Work out the finished part from the listing and answer in its coordinate system (mm). A direction names the side the tool comes from. Coordinates: 2 decimals unless noted, no trailing zeros. Loops run counter-clockwise (first coordinate to the right, second up) from the corner with the lowest first, then second, coordinate; pieces in that order, holes last. Notation, with made-up numbers: (70, -22.75) -> (84, -22.75) arc R24 ccw to (84, 7.25) -> close; hole circle Ø11 at (73.25, 47). An arc over 180 degrees is marked (long way). Answer as CSV lines item,"result".
```python
from build123d import *

# Parameters (mm, degrees)
DODANIE_WYCI_GNI_CIE1_DEPTH = 10
WYTNIJ_WYCI_GNI_CIE1_REACH  = 105.793
SZKIC2_R                    = 14
DODANIE_WYCI_GNI_CIE2_DEPTH = 450
DODANIE_WYCI_GNI_CIE3_DEPTH = 10
WYTNIJ_WYCI_GNI_CIE2_REACH  = 483.22
SZKIC5_R                    = 12.5
SZKIC7_W                    = 85
SZKIC7_H                    = 470
WYTNIJ_WYCI_GNI_CIE3_DEPTH  = 2
ZAOKR_GLENIE1_R             = 2
WYTNIJ_WYCI_GNI_CIE4_REACH  = 488.404
SZKIC8_W                    = 81
SZKIC8_H                    = 140
WYTNIJ_WYCI_GNI_CIE5_REACH  = 487.889
SZKIC9_W                    = 95
SZKIC9_H                    = 110


with BuildPart() as part:
    # Szkic1 → Dodanie-wyciągnięcie1 (new body)
    with BuildSketch(Plane.XY):
        Polygon((70, 47), (-70, 47), (-92, -40), (92, -40), align=None)
    extrude(amount=DODANIE_WYCI_GNI_CIE1_DEPTH)

    # Szkic2 → Wytnij-wyciągnięcie1 (cut, up to next)
    with BuildSketch(Plane(origin=(0, 0, 0), x_dir=(-1, 0, 0), z_dir=(0, 0, -1)), mode=Mode.PRIVATE) as wytnij_wyci_gni_cie1_sk1:
        Circle(SZKIC2_R)
    wytnij_wyci_gni_cie1_tool1 = extrude(wytnij_wyci_gni_cie1_sk1.sketch, amount=-WYTNIJ_WYCI_GNI_CIE1_REACH, mode=Mode.PRIVATE) & part.part
    add(wytnij_wyci_gni_cie1_tool1.solids().sort_by_distance((0, 0, 0))[0], mode=Mode.SUBTRACT)

    # Szkic3 → Dodanie-wyciągnięcie2 (add)
    with BuildSketch(Plane.XY.offset(10)):
        Polygon((-71.264367816, 42), (71.264367816, 42), (92, -40), (-92, -40), align=None)
        Polygon((-63.478332297, 32), (63.478332297, 32), (78.65074609, -28), (-78.65074609, -28), align=None, mode=Mode.SUBTRACT)
    extrude(amount=DODANIE_WYCI_GNI_CIE2_DEPTH)

    # Szkic4 → Dodanie-wyciągnięcie3 (add)
    with BuildSketch(Plane.XY.offset(460)):
        Polygon((-70, 47), (-92, -40), (92, -40), (70, 47), align=None)
    extrude(amount=DODANIE_WYCI_GNI_CIE3_DEPTH)

    # Szkic5 → Wytnij-wyciągnięcie2 (cut, up to next)
    with BuildSketch(Plane.XY.offset(470), mode=Mode.PRIVATE) as wytnij_wyci_gni_cie2_sk1:
        Circle(SZKIC5_R)
    wytnij_wyci_gni_cie2_tool1 = extrude(wytnij_wyci_gni_cie2_sk1.sketch, amount=-WYTNIJ_WYCI_GNI_CIE2_REACH, mode=Mode.PRIVATE) & part.part
    add(wytnij_wyci_gni_cie2_tool1.solids().sort_by_distance((0, 0, 470))[0], mode=Mode.SUBTRACT)

    # Szkic7 → Wytnij-wyciągnięcie3 (cut)
    with BuildSketch(Plane.XZ.offset(40)):
        with Locations((0, 235)):
            Rectangle(SZKIC7_W, SZKIC7_H)
    extrude(amount=-WYTNIJ_WYCI_GNI_CIE3_DEPTH, mode=Mode.SUBTRACT)

    # Zaokrąglenie1
    zaokr_glenie1_edges = [part.edges().sort_by_distance(p)[0] for p in [
        (42.5, -38, 235),
        (-42.5, -38, 235),
    ]]
    fillet(zaokr_glenie1_edges, radius=ZAOKR_GLENIE1_R - 0.0001)  # a hair under: the kernel refuses the full size

    # Szkic8 → Wytnij-wyciągnięcie4 (cut, up to next)
    with BuildSketch(Plane.XZ.offset(38), mode=Mode.PRIVATE) as wytnij_wyci_gni_cie4_sk1:
        with Locations((0, 235)):
            Rectangle(SZKIC8_W, SZKIC8_H)
    wytnij_wyci_gni_cie4_tool1 = extrude(wytnij_wyci_gni_cie4_sk1.sketch, amount=-WYTNIJ_WYCI_GNI_CIE4_REACH, mode=Mode.PRIVATE) & part.part
    add(wytnij_wyci_gni_cie4_tool1.solids().sort_by_distance((0, -38, 235))[0], mode=Mode.SUBTRACT)

    # Szkic9 → Wytnij-wyciągnięcie5 (cut, up to next)
    with BuildSketch(Plane(origin=(0, 42, 0), x_dir=(1, 0, 0), z_dir=(0, 1, 0)), mode=Mode.PRIVATE) as wytnij_wyci_gni_cie5_sk1:
        with Locations((0.805940964, -235)):
            Rectangle(SZKIC9_W, SZKIC9_H)
    wytnij_wyci_gni_cie5_tool1 = extrude(wytnij_wyci_gni_cie5_sk1.sketch, amount=-WYTNIJ_WYCI_GNI_CIE5_REACH, mode=Mode.PRIVATE) & part.part
    add(wytnij_wyci_gni_cie5_tool1.solids().sort_by_distance((0.805941, 42, 235))[0], mode=Mode.SUBTRACT)


solid = part.part
```
(1) Consider line 1 along Z through (x, y) = (52.5, 4); line 2 along Y through (x, z) = (-54, 299.5); line 3 along Y through (x, z) = (0, 5.75). Determine where each line is inside the solid, lowest interval first.
Computed values:
line 1,"0 to 10, 460 to 470"
line 2,"-40 to -28, 32 to 42"
line 3,"-38 to -14, 14 to 47"
(2) A cutting plane is placed at B-B, the plane x = 0. Write down the section's boundary in (y, z), and give its area (3 significant figures).
Computed values:
outline,"(-38, 0) -> (-14, 0) -> (-14, 10) -> (-28, 10) -> (-28, 165) -> (-38, 165) -> close; (-38, 305) -> (-28, 305) -> (-28, 460) -> (-12.5, 460) -> (-12.5, 470) -> (-38, 470) -> close; (12.5, 460) -> (32, 460) -> (32, 290) -> (42, 290) -> (42, 460) -> (47, 460) -> (47, 470) -> (12.5, 470) -> close; (14, 0) -> (47, 0) -> (47, 10) -> (42, 10) -> (42, 180) -> (32, 180) -> (32, 10) -> (14, 10) -> close"
area,"7,670 mm2"
(3) A cutting plane is placed at D-D, the plane y = 0. Write down the section's boundary in (x, z).
Computed values:
outline,"(-81.89, 0) -> (-14, 0) -> (-14, 10) -> (-71.57, 10) -> (-71.57, 460) -> (-12.5, 460) -> (-12.5, 470) -> (-81.89, 470) -> close; (12.5, 460) -> (71.57, 460) -> (71.57, 10) -> (14, 10) -> (14, 0) -> (81.89, 0) -> (81.89, 470) -> (12.5, 470) -> close"
(4) For a pull along Y with two mould halves and no side action, classify faces 5 (the face through (67, -40, 232)), 6 (the face through (-1, 14, 470)), 7 (the face through (70.96, 2.42, 231.85)), 8 (the face through (11.923, 3.755, 465.07)) as pulls with the +Y half, pulls with the -Y half, needs draft (parallel to the pull), parting line crosses it, or undercut.
Computed values:
face 5,"pulls with the -Y half"
face 6,"needs draft"
face 7,"undercut"
face 8,"undercut"
(5) Which of the six approach directions +Z, -Z, +X, -X, +Y, -Y give full straight-line access (tool end or side, diameter ignored) to faces 1 (the face through (48.306, 37, 236)), 2 (the face through (-1, -33, 305)), 3 (the face through (56, 32, 232)), 4 (the face through (-1, -38, 343))?
Computed values:
face 1,"+Y"
face 2,"-Y"
face 3,"none"
face 4,"+Z, -Z, -Y"
(6) Flat-ended cylindrical pins translate along their axes: pin 1 Ø6 at (x, y) = (59, 32.5) entering from -Z; pin 2 Ø3 at (y, z) = (-33.5, 259.5) entering from +X; pin 3 Ø5 at (y, z) = (28.5, 238) entering from +X; pin 4 Ø6 at (y, z) = (-12.5, 74) entering from +X. Find the tip coordinate at first contact, or state that the pin passes through.
Computed values:
pin 1,"z = 0"
pin 2,"x = 90.74"
pin 3,"x = 75.31"
pin 4,"x = 85.8"
